Can you work these out from the drawing? Everything is in mm from the part's minimum corner. A direction names the side the tool comes from. Give positions to 0.01 mm unless a question says otherwise; leave off trailing zeros. Loops run counter-clockwise (first coordinate to the right, second up) from the corner with the lowest first, then second, coordinate; pieces in that order, holes last. Notation, with made-up numbers: (-21, -15) -> (-10, -15) arc R19 ccw to (-10, 19) -> close; hole circle Ø5 at (75.25, -36.5). An arc over 180 degrees is marked (long way). Return JSON: item names as keys, results as strings. Group by question number.
Q1. Suppose I cut it at B-B, the plane z = 4. Please give me the cut outline in (x, y), and give its area (3 significant figures).
Q2. Will these pins go through, and if not, where does the flat tip stop? pin 1 (4 mm diameter, centred on x = 29.5, y = 14.5, fed in from +Z); pin 2 (0.6 mm diameter, centred on x = 8.5, y = 5, fed in from +Z).
Q3. Thinking about a two-plate mould opening in X: for the marked faces 1, 2 and 3, which applies, pulls with the +X half, pulls with the -X half, needs draft (parallel to the pull), parting line crosses it, or undercut?
Q4. Suppose I cut it at D-D, the plane y = 9.75. Please give me the cut outline in (x, z), and give its area (3 significant figures).
Q5. I need wall thicknesses on line 1 along Y through (x, z) = (8.5, 7.75); line 2 along X through (y, z) = (8, 8.25); line 3 along Y through (x, z) = (25, 10.25). Which ranges of each line are inside material? Lowest first, please. Write a range as [from, to].
Q6. Suppose I cut it at A-A, the plane z = 9.25. Please give me the cut outline in (x, y).
Q7. Suppose I cut it at C-C, the plane x = 38.5. Please give me the cut outline in (y, z), and give its area (4 significant figures).
Q8. Which directions (+Z, -Z, +X, -X, +Y, -Y) give clear straight access to the entire face, cutting with the end or side of a thin tool? Please do the marked faces 4 and 5.
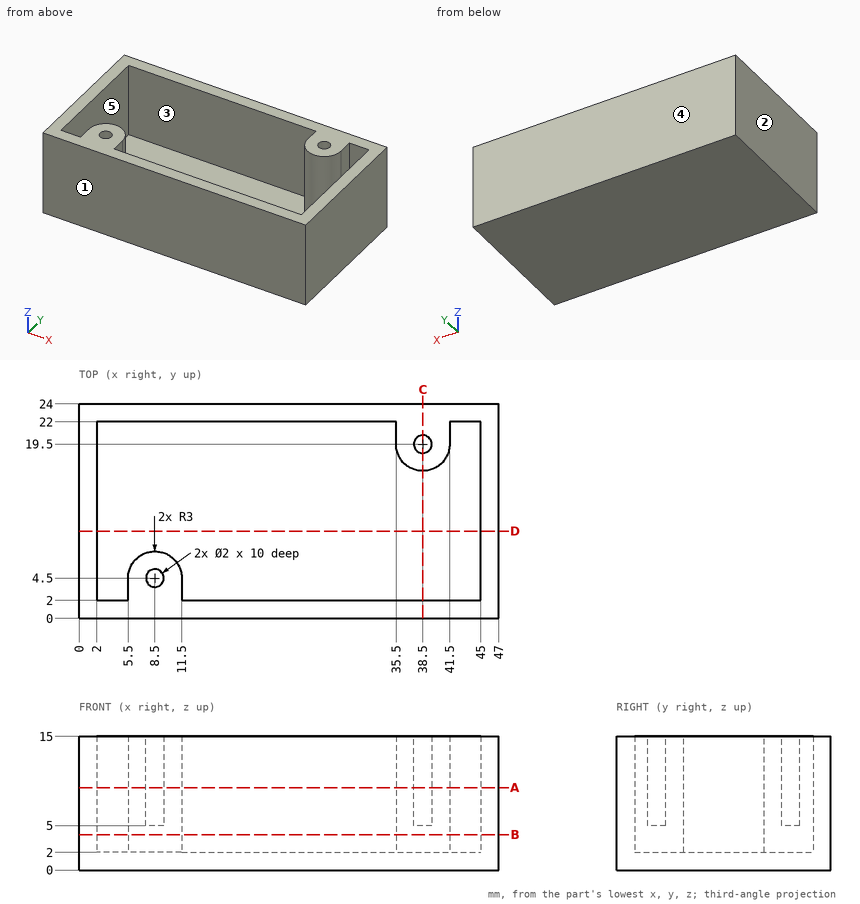
Ans:
{
 "1": {"outline": "(0, 0) -> (47, 0) -> (47, 24) -> (0, 24) -> close; hole (2, 2) -> (5.5, 2) -> (5.5, 4.5) arc R3 cw to (11.5, 4.5) -> (11.5, 2) -> (45, 2) -> (45, 22) -> (41.5, 22) -> (41.5, 19.5) arc R3 cw to (35.5, 19.5) -> (35.5, 22) -> (2, 22) -> close", "area": "326 mm^2"},
 "2": {"pin 1": "stops at z = 2", "pin 2": "stops at z = 5"},
 "3": {"face 1": "needs draft", "face 2": "pulls with the -X half", "face 3": "undercut"},
 "4": {"outline": "(0, 0) -> (47, 0) -> (47, 15) -> (45, 15) -> (45, 2) -> (2, 2) -> (2, 15) -> (0, 15) -> close", "area": "146 mm^2"},
 "5": {"line 1": "y = [0, 3.5], [5.5, 7.5], [22, 24]", "line 2": "x = [0, 2], [45, 47]", "line 3": "y = [0, 2], [22, 24]"},
 "6": {"outline": "(0, 0) -> (47, 0) -> (47, 24) -> (0, 24) -> close; hole (2, 2) -> (5.5, 2) -> (5.5, 4.5) arc R3 cw to (11.5, 4.5) -> (11.5, 2) -> (45, 2) -> (45, 22) -> (41.5, 22) -> (41.5, 19.5) arc R3 cw to (35.5, 19.5) -> (35.5, 22) -> (2, 22) -> close; hole circle Ø2 at (8.5, 4.5); hole circle Ø2 at (38.5, 19.5)"},
 "7": {"outline": "(0, 0) -> (24, 0) -> (24, 15) -> (20.5, 15) -> (20.5, 5) -> (18.5, 5) -> (18.5, 15) -> (16.5, 15) -> (16.5, 2) -> (2, 2) -> (2, 15) -> (0, 15) -> close", "area": "151.5 mm^2"},
 "8": {"face 4": "+Z, -Z, +X, -X, +Y", "face 5": "+Z"}
}
